CAD build for the part. Positions are in the model's coordinates, mm. Coordinates: 2 decimals unless noted, no trailing zeros. Loops run counter-clockwise (first coordinate to the right, second up) from the corner with the lowest first, then second, coordinate; pieces in that order, holes last.
1) Saw through at A-A, the plane z = 513.5. Write the cut outline in (x, y), and give its area (3 significant figures).
2) Wall check: line 1 along Z through (x, y) = (0, -13.3) (3 decimals); line 2 along Y through (x, z) = (2.25, 475.5); line 3 along Y through (x, z) = (-2.5, 75). Give the ranges that are in metal, low to high.
3) Pin check, flat tips, straight feed: pin 1 Ø1.5 at (x, z) = (6, 362) entering from +Y; pin 2 Ø8 at (x, z) = (5, 957.5) entering from -Y; pin 3 Ø10 at (y, z) = (-9, 574.5) entering from +X. Stop position of each tip, or through.
4) Two-plate mould, pull along Y, no slides. Class faces 1 (the cylindrical face through (10.902, -3.433, 601.066)), 2 (the cylindrical face through (-1.82, -13.85, 601.07)), 3 (the flat face through (-11.4, 2.1, 0)): +Y half, -Y half, draft (parallel to the pull), parting line (faces both ways), or undercut.
Autodesk Inventor part; units mm, degrees
ref_plane "Work Plane3" through (13.97, 0, 0) normal (1, 0, 0) x (0, 1, 0)
ref_plane "Work Plane4" through (0, 13.97, 0) normal (0, 1, 0) x (-1, 0, 0)
ref_plane "XY Plane" through (0, 0, 0) normal (0, 0, 1) x (1, 0, 0)
sketch "Sketch1" plane through (0, 0, 0) normal (0, 0, 1) x (1, 0, 0)
  circle A0 centre (0, 0) radius 11.43
  circle A1 centre (0, 0) radius 13.97
  dimension "d0" = 27.94
  dimension "d1" = 22.86
extrude "Extrusion1" add sketch "Sketch1" along normal blind 1219.2
ref_plane "Work Plane3" through (13.97, 0, 0) normal (1, 0, 0) x (0, 1, 0)
sketch "Sketch3" plane through (13.97, 0, 0) normal (1, 0, 0) x (0, 1, 0)
  circle A0 centre (0, 1092.2) radius 3.175
  line L0 (13.97, 1219.2) -> (-13.97, 1219.2)
  point P0 (0, 0)
  dimension "d5" = 127
  dimension "d6" = 6.35
extrude "Extrusion2" cut sketch "Sketch3" against normal through all
ref_plane "Work Plane4" through (0, 13.97, 0) normal (0, 1, 0) x (-1, 0, 0)
sketch "Sketch4" plane through (0, 13.97, 0) normal (0, 1, 0) x (-1, 0, 0)
  circle A0 centre (0, 1193.8) radius 3.175
  line L0 (13.97, 1219.2) -> (-13.97, 1219.2)
  point P0 (0, 0)
  dimension "d9" = 6.35
  dimension "d10" = 25.4
extrude "Extrusion3" cut sketch "Sketch4" against normal through all
equation "\"d1\" = cArmInsideDiam"
equation "\"d5\" = cArmAxelDistanceFromEnd"
equation "\"d6\" = boltHolesDiam"
equation "\"d9\" = boltHolesDiam"
equation "\"d10\" = cArmHingeDistanceFromEnd"
equation "\"cArmAxelDistanceFromEnd\" = 127"
equation "\"cArmOutsideDiam\" = 27.94"
equation "\"cArmInsideDiam\" = 22.86"
equation "\"cArmLength\" = 1219.2"
equation "\"boltHolesDiam\" = 6.35"
equation "\"cArmHingeDistanceFromEnd\" = 25.4"
properties part number "roundCatapultArm"
Data:
1. outline: circle Ø27.94 at (0, 0); hole circle Ø22.86 at (0, 0)
1. area: 203 mm2
2. line 1: z = 0 to 1190.625, 1196.975 to 1219.2
2. line 2: y = -13.79 to -11.21, 11.21 to 13.79
2. line 3: y = -13.74 to -11.15, 11.15 to 13.74
3. pin 1: stops at y = 12.95
3. pin 2: stops at y = -13.93
3. pin 3: stops at x = 13.39
4. face 1: undercut
4. face 2: parting line
4. face 3: draft
